Design review of the part built by this model. Coordinates are the model's own, in mm. Face numbers are marked on the shaded views. Round coordinates to 2 decimals unless told otherwise and drop trailing zeros. Loops run counter-clockwise (first coordinate to the right, second up) from the corner with the lowest first, then second, coordinate; pieces in that order, holes last. Notation, with made-up numbers: (31.25, -6.5) - (83.25, -6.5) arc R17 cw to (83.25, 15.5) - close; hole circle Ø10 at (-7.5, 66.5). An arc over 180 degrees is marked (long way). Return JSON: item names as keys, results as strings. Group by question number.
(1) We need section B-B, the plane z = 0.5. Give the number of separate pieces and of enclosed holes in the cut face, and give its area (3 significant figures).
(2) Wall thickness on L1, parallel to Y at x = 10, z = 1.2; L2, parallel to X at y = -11.25, z = 4.65; L3, parallel to X at y = -10.5, z = 0.75: over which ranges is each line inside the solid? List them lowest first. Write a range as [from, to].
(3) The part is to be moulded in two halves that separate along X. For the marked faces 1, 2 and 3, say which applies: pulls with the +X half, pulls with the -X half, needs draft (parallel to the pull), parting line crosses it, or undercut.
(4) We need section A-A, the plane x = 10. Write out the cut boundary in (y, z).
(5) Clearance check with flat-ended pins moving along their axes: pin 1 (1.5 mm diameter, centred on x = 6, z = 0.5, fed in from +Y); pin 2 (1 mm diameter, centred on y = -10.5, z = 4, fed in from +X); pin 3 (3.5 mm diameter, centred on x = 20, y = -10, fed in from -Z). State where each tip first meets the part, or that it passes through.
from build123d import *

# Parameters (mm, degrees)
SKETCH1_W           = 30
SKETCH1_H           = 13
BOSS_EXTRUDE1_DEPTH = 5
SKETCH2_R           = 1.6
CUT_EXTRUDE1_DEPTH  = 34.075670817
FILLET1_R           = 8
FILLET_2_R          = 6
CHAMFER_1_SIZE      = 0.2


with BuildPart() as part:
    # Sketch1 → Boss-Extrude1 (new body)
    with BuildSketch(Plane.XY):
        with Locations((15, -6.5)):
            Rectangle(SKETCH1_W, SKETCH1_H)
    extrude(amount=BOSS_EXTRUDE1_DEPTH)

    # Sketch2 → Cut-Extrude1 (cut, through all)
    with BuildSketch(Plane(origin=(0, 0, 0), x_dir=(-1, 0, 0), z_dir=(0, 0, -1))):
        with Locations((-20, -10)):
            Circle(SKETCH2_R)
        with Locations((-10, -10)):
            Circle(SKETCH2_R)
    extrude(amount=-CUT_EXTRUDE1_DEPTH, mode=Mode.SUBTRACT)

    # Fillet1
    # the kernel refuses this fillet: 8 mm, written as the material it takes off along each edge
    with BuildSketch(Plane(origin=(0, 0, -20), x_dir=(1, 0, 0), z_dir=(0, 0, 1)), Plane(origin=(0, -13, -20), x_dir=(0, 1, 0), z_dir=(0, 0, 1))) as fillet1_piece_1:
        with BuildLine():
            CenterArc((FILLET1_R, -FILLET1_R), FILLET1_R, 90, 90)
            Line((0, -FILLET1_R), (0, 0))
            Line((0, 0), (FILLET1_R, 0))
        make_face()
    extrude(amount=45, mode=Mode.SUBTRACT)
    with BuildSketch(Plane(origin=(30, -13, -20), x_dir=(0, 1, 0), z_dir=(0, 0, 1)), Plane(origin=(30, 0, -20), x_dir=(-1, 0, 0), z_dir=(0, 0, 1))) as fillet1_piece_2:
        with BuildLine():
            CenterArc((FILLET1_R, FILLET1_R), FILLET1_R, 180, 90)
            Line((0, FILLET1_R), (0, 0))
            Line((0, 0), (FILLET1_R, 0))
        make_face()
    extrude(amount=45, mode=Mode.SUBTRACT)

    # 圆角2
    fillet_2_edges = [part.edges().sort_by_distance(p)[0] for p in [
        (0.141883177, -6.5, 2.5),
        (29.858116823, -6.5, 2.5),
    ]]
    fillet(fillet_2_edges, radius=FILLET_2_R)

    # 倒角1
    chamfer_1_edges = [part.edges().sort_by_distance(p)[0] for p in [
        (21.6, -10, 5),
        (21.6, -10, 0),
        (11.6, -10, 5),
        (11.6, -10, 0),
        (15, 0, 0),
        (15, -13, 0),
        (24.828427125, -0.516685226, 0),
        (5.171572875, -12.483314774, 0),
        (15, 0, 5),
        (15, -13, 5),
        (24.828427125, -12.483314774, 5),
        (5.171572875, -0.516685226, 5),
        (24.828427125, -12.483314774, 0),
        (5.171572875, -12.483314774, 5),
        (24.828427125, -0.516685226, 5),
        (0.677124344, -6.5, 5),
        (29.322875656, -6.5, 5),
        (5.171572875, -0.516685226, 0),
        (0.677124344, -6.5, 0),
        (29.322875656, -6.5, 0),
    ]]
    chamfer(chamfer_1_edges, length=CHAMFER_1_SIZE)


solid = part.part
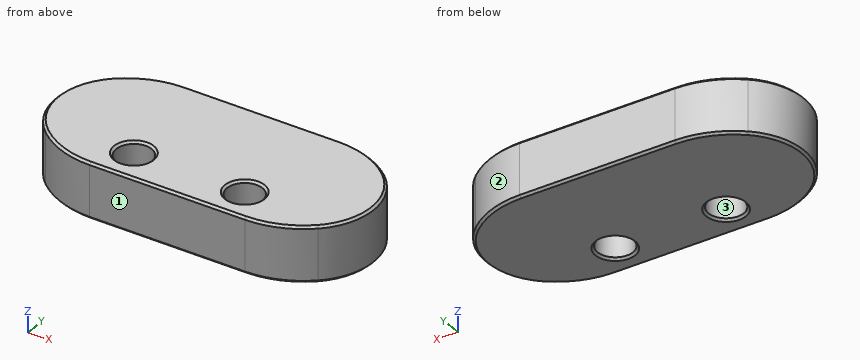
Solutions:
{
 "1": {"separate pieces": "1", "enclosed holes": "2", "area": "316 mm^2"},
 "2": {"L1": "[-13, -11.6], [-8.4, 0]", "L2": "[3.01, 9], [11, 19], [21, 26.99]", "L3": "[2.2, 8.48], [11.52, 18.48], [21.52, 27.8]"},
 "3": {"face 1": "needs draft", "face 2": "pulls with the +X half", "face 3": "undercut"},
 "4": {"outline": "(-13, 0.2) - (-12.8, 0) - (-11.8, 0) - (-11.6, 0.2) - (-11.6, 4.8) - (-11.8, 5) - (-12.8, 5) - (-13, 4.8) - close; (-8.4, 0.2) - (-8.2, 0) - (-0.2, 0) - (0, 0.2) - (0, 4.8) - (-0.2, 5) - (-8.2, 5) - (-8.4, 4.8) - close"},
 "5": {"pin 1": "y = -0.1", "pin 2": "x = 28.2", "pin 3": "z = 0.05"}
}
